Could you check a few things on this drawing? It's one solid part, dimensions in mm from its lowest x, y, z. A direction names the side the tool comes from. Give positions to 0.01 mm unless a question says otherwise; leave off trailing zeros. Order: outer loops, then holes, each group sorted by start corner. A loop starts at its lowest first (then second) coordinate and runs counter-clockwise, first axis right, second up. Notation, with made-up numbers: (47, -19.5) -> (98, -19.5) arc R13 ccw to (98, -9.5) -> close; hole circle Ø4 at (-39, 53). An arc over 180 degrees is marked (long way). Answer as a JSON object with one key per item and string values.
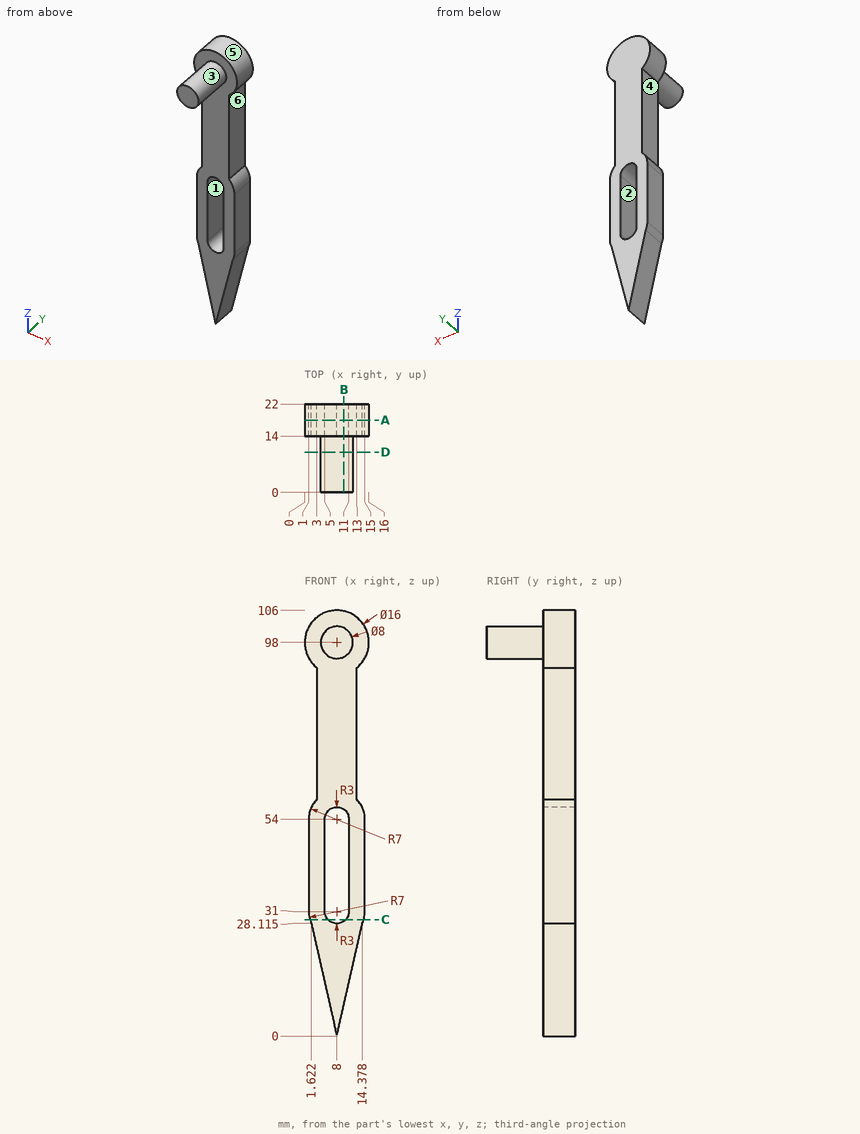
1. If we section it at D-D on y = 10: Please give me the cut outline in (x, z).
Worked answers:
{"outline": "circle Ø8 at (8, 98)"}
2. If we section it at B-B on x = 9.75: Please give me the cut outline in (y, z) (1 decimal).
Worked answers:
{"outline": "(0, 94.4) -> (14, 94.4) -> (14, 56.4) -> (22, 56.4) -> (22, 105.8) -> (14, 105.8) -> (14, 101.6) -> (0, 101.6) -> close; (14, 7.7) -> (22, 7.7) -> (22, 28.6) -> (14, 28.6) -> close"}
3. Please list where these lines run through material, in increasing order: L1, parallel to X at y = 16, z = 50.5; L2, parallel to Y at x = 9.5, z = 83; L3, parallel to Z at x = 7.75, y = 5.25.
Worked answers:
{"L1": "1 to 5, 11 to 15", "L2": "14 to 22", "L3": "94.01 to 101.99"}
4. If we mould it in two halves opening along X, with no side actions, what happens to the marked faces 1, 2, 3 and 4? For each: +X half, -X half, draft (parallel to the pull), parting line (faces both ways), or undercut.
Worked answers:
{"face 1": "undercut", "face 2": "undercut", "face 3": "parting line", "face 4": "-X half"}
5. If we section it at A-A on y = 18: Please give me the cut outline in (x, z) (1 decimal).
Worked answers:
{"outline": "(1, 31) arc R7 ccw to (1.6, 28.1) -> (8, 0) -> (14.4, 28.1) arc R7 ccw to (15, 31) -> (15, 54) arc R7 ccw to (13, 58.9) -> (13, 91.8) arc R8 ccw (long way) to (3, 91.8) -> (3, 58.9) arc R7 ccw to (1, 54) -> close; hole (5, 31) arc R3 ccw to (11, 31) -> (11, 54) arc R3 ccw to (5, 54) -> close"}
6. Will these pins go through, and if not, where does the flat tip stop? pin 1 Ø4 at (y, z) = (17, 82) entering from +X; pin 2 Ø6.5 at (y, z) = (20, 46) entering from +X; pin 3 Ø6 at (x, y) = (6, 15) entering from +Z; pin 4 Ø6.5 at (y, z) = (18, 75) entering from -X.
Worked answers:
{"pin 1": "x = 13", "pin 2": "x = 15", "pin 3": "z = 106", "pin 4": "x = 3"}
7. If we section it at C-C on z = 29: Please give me the cut outline in (x, y).
Worked answers:
{"outline": "(1.29, 14) -> (5.76, 14) -> (5.76, 22) -> (1.29, 22) -> close; (10.24, 14) -> (14.71, 14) -> (14.71, 22) -> (10.24, 22) -> close"}
8. For the marked faces 5 and 6, which set-ups out of +Z, -Z, +X, -X, +Y, -Y let a thin tool reach every point of the face, with its end or its side?
Worked answers:
{"face 5": "+Y, -Y", "face 6": "+X, +Y, -Y"}
